from build123d import *

# Parameters (mm, degrees)
F0_R     = 1.5
F1_DEPTH = 7
F2_R     = 1
F3_R     = 1


with BuildPart() as f1:
    # F0 (on Top) → F1 (new body)
    with BuildSketch(Plane.XY):
        with BuildLine():
            Line((-51.473763, -12.437916), (-1.742005, -17.413082))
            ThreePointArc((-1.742005, -17.413082), (17.5, 0), (-1.742005, 17.413082))
            Line((-1.742005, 17.413082), (-51.473763, 12.437916))
            ThreePointArc((-51.473763, 12.437916), (-62.729473, 0), (-51.473763, -12.437916))
        make_face()
        Polygon((4.907477, 8.5), (9.814955, 0), (4.907477, -8.5), (-4.907477, -8.5), (-5.196152, -8), (-14.433757, -8), (-14.722432, -7.5), (-23.382686, -7.5), (-23.671361, -7), (-31.754265, -7), (-32.04294, -6.5), (-39.548493, -6.5), (-39.837169, -6), (-46.765372, -6), (-47.054047, -5.5), (-53.4049, -5.5), (-56.580326, 0), (-53.4049, 5.5), (-47.054047, 5.5), (-46.765372, 6), (-39.837169, 6), (-39.548493, 6.5), (-32.04294, 6.5), (-31.754265, 7), (-23.671361, 7), (-23.382686, 7.5), (-14.722432, 7.5), (-14.433757, 8), (-5.196152, 8), (-4.907477, 8.5), align=None, mode=Mode.SUBTRACT)
        with Locations((13.5, 0)):
            Circle(F0_R, mode=Mode.SUBTRACT)
    extrude(amount=F1_DEPTH)

    # F2
    f2_edges = [f1.edges().sort_by_distance(p)[0] for p in [
        (-62.729473, 0, 7),
        (-26.607884, -14.925499, 0),
    ]]
    fillet(f2_edges, radius=F2_R)

    # F3
    f3_edges = [f1.edges().sort_by_distance(p)[0] for p in [
        (12, 0, 7),
        (12, 0, 0),
    ]]
    fillet(f3_edges, radius=F3_R)


solid = f1.part
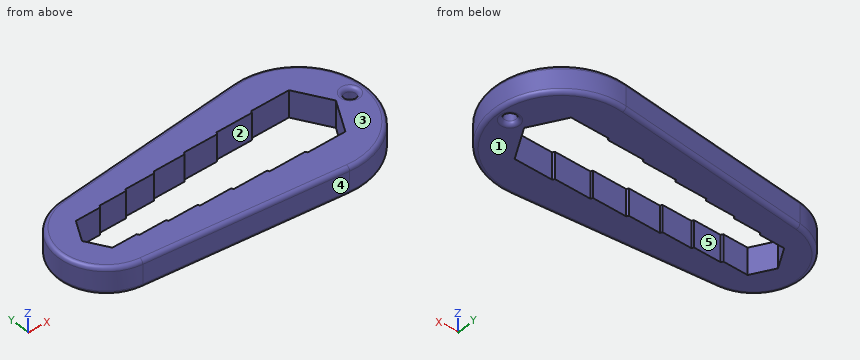
Geometry: final body of the model. Coordinates: model frame, mm. Face numbers are marked on the shaded views. A direction names the side the tool comes from. Round coordinates to 2 decimals unless told otherwise and drop trailing zeros. Put each result on its own line as item: value. Start each with the question number.
Q1. Line query: probe 1 along Y at (x, z) = (0, 5); probe 2 along X at (y, z) = (-4, 0.5); probe 3 along Y at (x, z) = (-3, 6). Output: solid intervals per line, ascending.
Q2. First-contact query: pin 1 (4 mm diameter, centred on y = -14, z = 3, fed in from +X); pin 2 (2 mm diameter, centred on y = 3.5, z = 3.5, fed in from +X); pin 3 (3 mm diameter, centred on x = 5.5, y = -7, fed in from +Z); pin 4 (1 mm diameter, centred on y = 9, z = 1.5, fed in from -X). Flat tips, straight axial feed; report the tip coordinate or a pass-through.
Q3. Pull-direction query (X, two-part tool) for the marked faces 3, 4 and 5; classes: +X half, -X half, draft (parallel to the pull), parting line (faces both ways), or undercut.
Q4. Reachability of the marked faces 1 and 2 from +Z, -Z, +X, -X, +Y, -Y: full face, straight path, thin tool, end or side. Return the list, or none.
Q5. Section A-A on z = 3.25. Give the number of separate pieces and of enclosed holes in the cut face, and give its area (3 significant figures).
Ans:
1. probe 1: y = -17.5 to -8.5, 8.5 to 17.5
1. probe 2: x = -61.93 to -54.27, 7.51 to 16.9
1. probe 3: y = -17.29 to -8.5, 8.5 to 17.29
2. pin 1: stops at x = 12.74
2. pin 2: stops at x = 17.32
2. pin 3: stops at z = 7
2. pin 4: stops at x = -59.39
3. face 3: draft
3. face 4: -X half
3. face 5: undercut
4. face 1: -Z, +X, -X, +Y, -Y
4. face 2: +Z, -Z
5. separate pieces: 1
5. enclosed holes: 2
5. area: 1,340 mm2
